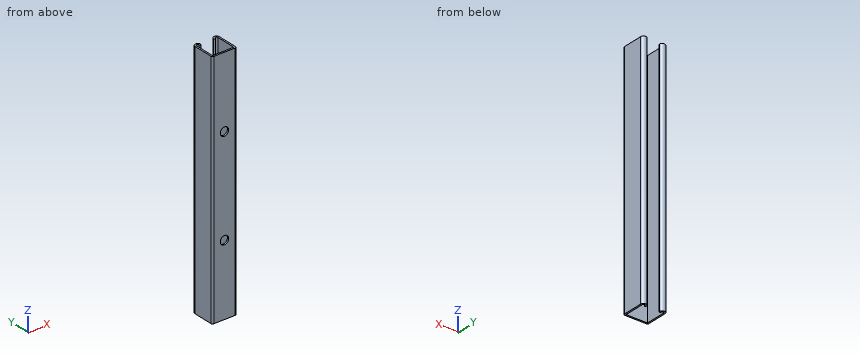
```python
from build123d import *

# Parameters (mm, degrees)
EXTRUDE_1_DEPTH     = 406.4
SKETCH_2_R          = 7.112
CUT_EXTRUDE_1_DEPTH = 411.319677278


with BuildPart() as part:
    # 草图1 → 凸台-拉伸1 (new body)
    with BuildSketch(Plane.XY):
        with BuildLine():
            Line((0, 0), (35.98, 0))
            ThreePointArc((35.98, 0), (37.883814298, 0.788585702), (38.6724, 2.6924))
            Line((38.6724, 2.6924), (38.6724, 36.5252))
            ThreePointArc((38.6724, 36.5252), (33.8972, 41.3004), (29.122, 36.5252))
            ThreePointArc((29.122, 36.5252), (30.4682, 35.179), (31.8144, 36.5252))
            ThreePointArc((31.8144, 36.5252), (33.8972, 38.608), (35.98, 36.5252))
            Line((35.98, 36.5252), (35.98, 2.6924))
            Line((35.98, 2.6924), (0, 2.6924))
            Line((0, 2.6924), (0, 36.5252))
            ThreePointArc((0, 36.5252), (2.0828, 38.608), (4.1656, 36.5252))
            ThreePointArc((4.1656, 36.5252), (5.5118, 35.179), (6.858, 36.5252))
            ThreePointArc((6.858, 36.5252), (2.0828, 41.3004), (-2.6924, 36.5252))
            Line((-2.6924, 36.5252), (-2.6924, 2.6924))
            ThreePointArc((-2.6924, 2.6924), (-1.903814298, 0.788585702), (0, 0))
        make_face()
    extrude(amount=EXTRUDE_1_DEPTH)

    # 草图2 → 切除-拉伸1 (cut, through all)
    with BuildSketch(Plane(origin=(0, 0, 0), x_dir=(-1, 0, 0), z_dir=(0, -1, 0))):
        with Locations(Location((-17.99, -120.65, 0), (0, 0, 90))):
            Circle(SKETCH_2_R)
        with Locations(Location((-17.99, -285.75, 0), (0, 0, 90))):
            Circle(SKETCH_2_R)
    extrude(amount=-CUT_EXTRUDE_1_DEPTH, mode=Mode.SUBTRACT)


solid = part.part
```
Read the model definition and answer for the solid it produces. Units are mm, in the model's axes. Coordinates: 2 decimals unless noted, no trailing zeros. Order: outer loops, then holes, each group sorted by start corner. A loop starts at its lowest first (then second) coordinate and runs counter-clockwise, first axis right, second up. Notation, with made-up numbers: (24, 2.5) - (58, 2.5) arc R27 ccw to (58, 20.5) - close; hole circle Ø11 at (-25, -15.5). An arc over 180 degrees is marked (long way). Answer as a JSON object with one key per item and string values. Group by question number.
Item 1: Section C-C (x = 17.99) is taken. Give the vertices of the cut face in (y, z), plus the area to 3 significant figures.
Item 2: Flat-ended cylindrical pins translate along their axes: P1, Ø18, axis at x = 12.5, z = 235.5, coming from the +Y side; P2, Ø1.5, axis at x = 17, z = 208, coming from the +Y side; P3, Ø16.5, axis at x = 17.99, z = 120.65, coming from the -Y side. Find the tip coordinate at first contact, or state that the pin passes through.
Item 3: Section A-A (y = 13) is taken. Give the vertices of the cut face in (x, z), plus the area to 3 significant figures.
Item 4: Consider probe 1 along X at (y, z) = (13.5, 198); probe 2 along X at (y, z) = (36, 176); probe 3 along Y at (x, z) = (19, 141). Determine where each line is inside the solid, lowest interval first. Write a range as from..to.
Results are:
{
 "1": {"outline": "(0, 0) - (2.69, 0) - (2.69, 113.54) - (0, 113.54) - close; (0, 127.76) - (2.69, 127.76) - (2.69, 278.64) - (0, 278.64) - close; (0, 292.86) - (2.69, 292.86) - (2.69, 406.4) - (0, 406.4) - close", "area": "1,020 mm^2"},
 "2": {"P1": "stops at y = 41.09", "P2": "stops at y = 2.69", "P3": "stops at y = 0"},
 "3": {"outline": "(-2.69, 0) - (0, 0) - (0, 406.4) - (-2.69, 406.4) - close; (35.98, 0) - (38.67, 0) - (38.67, 406.4) - (35.98, 406.4) - close", "area": "2,190 mm^2"},
 "4": {"probe 1": "x = -2.69..0, 35.98..38.67", "probe 2": "x = -2.69..0, 4.27..6.75, 29.23..31.71, 35.98..38.67", "probe 3": "y = 0..2.69"}
}
